Autodesk Inventor part; units mm, degrees
ref_plane "YZ Plane" through (0, 0, 0) normal (1, 0, 0) x (0, 1, 0)
ref_plane "XZ Plane" through (0, 0, 0) normal (0, 1, 0) x (-1, 0, 0)
ref_plane "XY Plane" through (0, 0, 0) normal (0, 0, 1) x (1, 0, 0)
sketch "スケッチ6" plane through (0, 0, 0) normal (0, 0, 1) x (1, 0, 0)
  circle A0 centre (0, 0) radius 13.5
  circle A1 centre (0, 0) radius 23.5
  circle A2 centre (-11.8916, -14.1718) radius 5
  line L0 (0, 0) -> (-11.8916, -14.1718)
  line L1 (0, 0) -> (0, -23.5)
  line L2 (13.5, 0) -> (63.5, 0)
  line L3 (63.5, 0) -> (63.5, -18)
  line L4 (63.5, -18) -> (13.5, -18)
  line L5 (13.5, -18) -> (13.5, 0)
  line L6 (48.5, 0) -> (63.5, 0)
  line L7 (63.5, 0) -> (63.5, -40)
  line L8 (63.5, -40) -> (48.5, -40)
  line L9 (48.5, -40) -> (48.5, 0)
  point P0 (-15.1055, -18.002)
  point P1 (48.5, -18)
  point P2 (-8.6776, -10.3416)
  point P3 (23.5, 0)
  point P4 (13.3373, -19.3486)
  point P5 (13.4479, -1.1846)
  point P6 (23.5, 0)
  point P7 (15.1079, -18)
  dimension "d31" = 27
  dimension "d32" = 47
  dimension "d33" = 10
  dimension "d34" = 40
  dimension "d35" = 50
  dimension "d36" = 18
  dimension "d37" = 15
  dimension "d38" = 0
  dimension "d63" = 40
extrude "押し出し4" add sketch "スケッチ6" along normal blind 6 contours L5 L4 A1 L1 A0 | L2 A1 L4 L5 | A0 L1 A1 A2 | A2 | L2 L9 L4 A1 | L2 L3 L4 L9 | L4 L7 L8 L9
sketch "スケッチ9" plane through (0, 0, 6) normal (0, 0, 1) x (1, 0, 0)
  line L0 (48.5, -40) -> (63.5, -40)
  line L1 (63.5, 0) -> (13.5, 0)
  point P0 (0, 0)
  point P1 (57.6485, -5)
  point P2 (57.6485, -35)
  dimension "d54" = 5
  dimension "d64" = 5
hole "穴4" at (57.6485, -5, 6) at (57.6485, -35, 6) direction (0, 0, -1) diameter 4.5 end through all
sketch "スケッチ10" plane through (0, 0, 0) normal (0, 0, -1) x (-1, 0, 0)
  circle A0 centre (-71, -7.5) radius 7.5
  line L0 (-63.5, -40) -> (-63.5, 0)
  line L1 (-63.5, 0) -> (-13.5, 0)
  line L2 (-63.5, -40) -> (-63.5, 0)
  line L3 (-71, 0) -> (-63.5, 0)
  line L4 (-63.5, 0) -> (-63.5, -15)
  line L5 (-63.5, -15) -> (-71, -15)
  line L6 (-71, -15) -> (-71, 0)
  point P0 (0, 0)
  dimension "d65" = 15
extrude "押し出し6" add sketch "スケッチ10" against normal blind 3
sketch "スケッチ11" plane through (0, 0, 3) normal (0, 0, 1) x (1, 0, 0)
  arc A0 (71, -15) -> (71, 0) centre (71, -7.5) ccw
  point P0 (0, 0)
hole "穴5" at (71, -7.5, 3) direction (0, 0, -1) diameter 4.5 end through all
sketch "スケッチ12" plane through (15.1079, -18, 0) normal (0, -1, 0) x (1, 0, 0)
  line L0 (-1.6079, 0) -> (55.8921, 0)
  line L1 (48.3921, 6) -> (-1.6079, 6)
  line L2 (20, 0) -> (15, 0)
  line L3 (15, 0) -> (15, 6)
  line L4 (15, 6) -> (20, 6)
  line L5 (20, 6) -> (20, 0)
  line L6 (0, 0) -> (0, 6)
  point P0 (-15.1079, 0)
  point P1 (15, 0)
  dimension "d75" = 5
  dimension "d82" = 15
extrude "押し出し7" add sketch "スケッチ12" along normal blind 6 contours L3 L1 L5 L0
sketch "スケッチ13" plane through (35.1079, -18, 6) normal (1, 0, 0) x (0, 0, -1)
  line L0 (6, 0) -> (0, 0)
  line L1 (0, 0) -> (2, 0)
  line L2 (2, 0) -> (2, -2)
  line L3 (2, -2) -> (0, -2)
  line L4 (0, -2) -> (0, 0)
  point P0 (6, 18)
  dimension "d78" = 2
  dimension "d79" = 2
extrude "押し出し8" cut sketch "スケッチ13" against normal blind 6
properties part number "エアタンクペットボトル取付具"
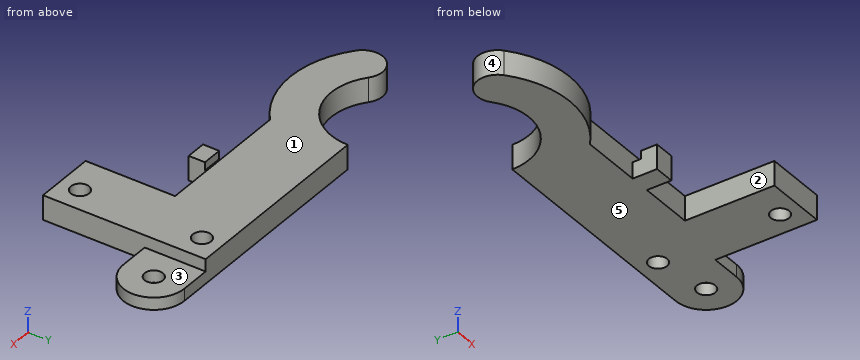
Can you work these out from the model? Positions are in its coordinate system, mm. Face numbers are marked on the shaded views. A direction names the side the tool comes from. Round coordinates to 2 decimals unless told otherwise and drop trailing zeros. Loops run counter-clockwise (first coordinate to the right, second up) from the corner with the lowest first, then second, coordinate; pieces in that order, holes last. Notation, with made-up numbers: M -25,14.25 L -14,14.25 A19 ccw -14,48.25 Z; hole C 31,53.25 d9. An arc over 180 degrees is marked long. Write item = value, one per line. Start each with the question number.
(1) I need wall thicknesses on line 1 along Y through (x, z) = (34, 4.1); line 2 along Y through (x, z) = (71, 1.8); line 3 along X through (y, z) = (-35, 4.5). Which ranges of each line are inside material? Lowest first, please.
(2) Suppose I cut it at A-A on y = -35. Write out the boundary of the cut face in (x, z).
(3) Which directions (+Z, -Z, +X, -X, +Y, -Y) give clear straight access to the entire face, cutting with the end or side of a thin tool? Please do the marked faces 1, 2 and 3.
(4) Suppose I cut it at B-B on x = 33. Write out the boundary of the cut face in (y, z), plus the area to 3 significant figures.
(5) Suppose I cut it at C-C on y = -12. Write out the boundary of the cut face in (x, z), plus the area to 3 significant figures.
(6) I'm going to push flat-ended pins straight in: P1, Ø1.5, axis at x = 35.5, z = 2, coming from the -Y side; P2, Ø3, axis at y = -21, z = 4, coming from the +X side; P3, Ø1.5, axis at y = -5, z = 1.5, coming from the -X side. Where does each tip first touch, or does it pass through?
(7) Suppose I cut it at D-D on y = -29.5. Write out the boundary of the cut face in (x, z), plus the area to 3 significant figures.
(8) If we mould it in two halves opening along X, with no side actions, what happens to the marked faces 4 and 5? For each: released by +X, released by -X, zero draft, split by the parting line, or undercut.
Answer block:
q1.line_1 = -24 to -20, -18 to 0
q1.line_2 = -15 to -9.75, -5.25 to 0
q1.line_3 = 48.5 to 55.4, 59.9 to 63.5
q2.outline = M 48.5,0 L 55.4,0 L 55.4,6 L 48.5,6 Z; M 59.9,0 L 63.5,0 L 63.5,6 L 59.9,6 Z
q3.face_1 = +Z, +X, -X, +Y, -Y
q3.face_2 = +Z, -Z, -Y
q3.face_3 = +Z, +X, +Y, -Y
q4.outline = M -24,0 L 0,0 L 0,6 L -18,6 L -18,4 L -20,4 L -20,6 L -24,6 Z
q4.area = 140 mm²
q5.outline = M -16.4,0 L -6.18,0 L -6.18,6 L -16.4,6 Z; M 6.18,0 L 77,0 L 77,3 L 63.5,3 L 63.5,6 L 6.18,6 Z
q5.area = 446 mm²
q6.P1 = -24
q6.P2 = 63.5
q6.P3 = 12.21
q7.outline = M 48.5,0 L 63.5,0 L 63.5,6 L 48.5,6 Z
q7.area = 90.0 mm²
q8.face_4 = undercut
q8.face_5 = zero draft
